Work out the finished part from the listing and answer in its coordinate system (mm). Face numbers are marked on the shaded views. A direction names the side the tool comes from. Round coordinates to 2 decimals unless told otherwise and drop trailing zeros. Order: outer loops, then holes, each group sorted by start corner. A loop starts at its lowest first (then second) coordinate and runs counter-clockwise, first axis right, second up. Notation, with made-up numbers: (27.25, 68.5) -> (38.25, 68.5) arc R20 cw to (38.25, 99.5) -> close; hole circle Ø6 at (-10.5, 87.25). An arc over 180 degrees is marked (long way). Use a Markdown table: item, result. Add a question column.
Item 1: Flat-ended cylindrical pins translate along their axes: P1, Ø6.5, axis at y = 44, z = 4, coming from the +X side; P2, Ø22.5, axis at x = 6.5, y = 19, coming from the -Z side; P3, Ø11, axis at y = 5.5, z = 5, coming from the +X side. Find the tip coordinate at first contact, or state that the pin passes through.
Item 2: A cutting plane is placed at C-C, the plane z = 2. Determine the outline of the cut face in (x, y), plus the area to 3 significant figures.
Item 3: For a pull along X with two mould halves and no side action, classify the marked faces 1, 2 and 3 as +X half, -X half, draft (parallel to the pull), parting line (faces both ways), or undercut.
Item 4: A tool of negligible diameter and unlimited length cuts with its end or side. For the marked faces 4, 5 and 6, from which of +Z, -Z, +X, -X, +Y, -Y can it reach the whole face along a straight path? Write none if from no direction.
Item 5: A cutting plane is placed at A-A, the plane y = 42. Give the number of separate pieces and of enclosed holes in the cut face, plus the area to 3 significant figures.
Item 6: A cutting plane is placed at B-B, the plane x = 65.75. Determine the outline of the cut face in (y, z).
Item 7: Find the intervals of material crossed by L1, parallel to Y at x = 65.75, z = -11; L2, parallel to Y at x = 10, z = -8.5; L3, parallel to X at y = 20, z = 7.25, in increasing order. Write a range as [from, to].
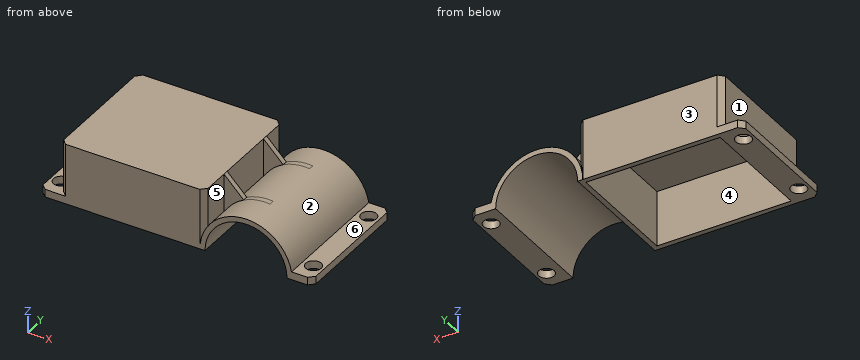
Autodesk Inventor part; units mm, degrees
ref_plane "YZ Plane" through (0, 0, 0) normal (1, 0, 0) x (0, 1, 0)
ref_plane "XZ Plane" through (0, 0, 0) normal (0, 1, 0) x (-1, 0, 0)
ref_plane "XY Plane" through (0, 0, 0) normal (0, 0, 1) x (1, 0, 0)
sketch "Esboço1" plane through (0, 0, 0) normal (0, 1, 0) x (-1, 0, 0)
  line L0 (-28, -11.75) -> (28, -11.75)
  line L1 (28, -11.75) -> (28, 11.75)
  line L2 (28, 11.75) -> (-28, 11.75)
  line L3 (-28, 11.75) -> (-28, -11.75)
  line L4 (-28, -11.75) -> (28, 11.75) construction
  line L5 (28, -11.75) -> (-28, 11.75) construction
  point P0 (0, 0)
  dimension "d0" = 56
  dimension "d1" = 23.5
extrude "Extrusão1" add sketch "Esboço1" along normal blind 49
sketch "Esboço2" plane through (28, 0, -11.75) normal (0, 0, -1) x (-1, 0, 0)
  line L0 (0, 49) -> (56, 49)
  line L1 (0, 49) -> (-33.75, 49)
  line L2 (-33.75, 49) -> (-33.75, 0)
  line L3 (0, 0) -> (56, 0)
  line L4 (-33.75, 0) -> (0, 0)
  line L5 (0, 0) -> (0, 49)
  point P0 (28, 0)
  dimension "d4" = 33.75
extrude "Extrusão2" add sketch "Esboço2" against normal blind 17.875
sketch "Esboço3" plane through (0, 49, 0) normal (0, 1, 0) x (1, 0, 0)
  line L0 (-28, 11.75) -> (61.75, 11.75)
  line L1 (61.75, 11.75) -> (59.75, 11.75)
  line L2 (59.75, 11.75) -> (43.875, 11.75)
  circle A0 centre (43.875, 11.75) radius 15.875
  point P0 (0, 0)
  dimension "d7" = 2
  dimension "d8" = 15.875
extrude "Extrusão3" cut sketch "Esboço3" against normal blind 49
sketch "Esboço4" plane through (61.75, 0, -11.75) normal (0, 0, -1) x (-1, 0, 0)
  line L0 (0, 49) -> (33.75, 49)
  line L1 (33.75, 0) -> (0, 0)
  line L2 (0, 49) -> (0, 0)
  line L3 (0, 0) -> (-8, 0)
  line L4 (-8, 0) -> (-8, 49)
  line L5 (-8, 49) -> (0, 49)
  line L6 (-4, 0) -> (-4, 7)
  line L7 (-4, 49) -> (-4, 42)
  circle A0 centre (-4, 42) radius 3
  circle A1 centre (-4, 7) radius 3
  point P0 (61.75, 0)
  dimension "d11" = 8
  dimension "d12" = 7
  dimension "d13" = 7
  dimension "d14" = 6
  dimension "d15" = 6
extrude "Extrusão4" add sketch "Esboço4" against normal blind 3
sketch "Esboço5" plane through (0, 49, 0) normal (0, 1, 0) x (1, 0, 0)
  arc A0 (28, 11.75) -> (59.75, 11.75) centre (43.875, 11.75) ccw
  circle A1 centre (43.875, 11.75) radius 17.875
  line L0 (61.75, -6.125) -> (28, -6.125)
  line L1 (69.75, 8.75) -> (61.75, 8.75)
  line L2 (61.75, 8.75) -> (61.4965, 8.75)
  line L3 (61.75, 8.75) -> (61.75, -6.125)
  line L4 (43.875, -6.125) -> (61.75, -6.125)
  line L5 (28, -11.75) -> (28, -6.125)
  line L6 (43.875, -6.125) -> (28, -6.125)
  line L7 (28, -6.125) -> (28, 3.5342)
  point P0 (0, 0)
extrude "Extrusão5" cut sketch "Esboço5" against normal blind 49 contours A1 L0 L7 | L2 L3 L0 A1
sketch "Esboço6" plane through (-28, 0, -11.75) normal (0, 0, -1) x (-1, 0, 0)
  line L0 (0, 0) -> (0, 49)
  line L1 (0, 49) -> (0, 0)
  line L2 (0, 0) -> (8, 0)
  line L3 (8, 0) -> (8, 49)
  line L4 (8, 49) -> (0, 49)
  line L5 (4, 49) -> (4, 42)
  line L6 (4, 0) -> (4, 7)
  circle A0 centre (4, 7) radius 3
  circle A1 centre (4, 42) radius 3
  point P0 (-28, 0)
  dimension "d20" = 8
  dimension "d21" = 7
  dimension "d22" = 7
  dimension "d23" = 6
  dimension "d24" = 6
extrude "Extrusão6" add sketch "Esboço6" against normal blind 3
sketch "Esboço8" plane through (28, 0, -11.75) normal (0, 0, -1) x (-1, 0, 0)
  line L0 (0, 49) -> (0, 0)
  line L1 (0, 49) -> (0, 47)
  line L2 (0, 47) -> (2, 47)
  line L3 (2, 47) -> (2, 2)
  line L4 (2, 47) -> (47, 47) construction
  line L5 (2, 2) -> (54, 2)
  line L6 (2, 2) -> (54, 2) construction
  line L7 (54, 2) -> (54, 47)
  line L8 (54, 47) -> (2, 47)
  point P0 (28, 0)
  dimension "d27" = 2
  dimension "d28" = 2
  dimension "d29" = 45
  dimension "d30" = 90
  dimension "d31" = 52
  dimension "d32" = 0
extrude "Extrusão7" cut sketch "Esboço8" against normal blind 21.5
sketch "Esboço10" plane through (28, 0, 11.75) normal (1, 0, 0) x (0, 0, -1)
  line L0 (0, 0) -> (0, 49)
  line L1 (0, 49) -> (0, 37)
  line L2 (0, 0) -> (0, 12)
  line L3 (0, 12) -> (16, 12)
  line L4 (16, 12) -> (16, 14)
  line L5 (16, 14) -> (0, 14)
  line L6 (0, 12) -> (0, 14)
  line L7 (0, 37) -> (16, 37)
  line L8 (16, 37) -> (16, 39)
  line L9 (16, 39) -> (0, 39)
  point P0 (11.75, 0)
  dimension "d38" = 12
  dimension "d41" = 12
  dimension "d42" = 16
  dimension "d43" = 2
  dimension "d44" = 16
  dimension "d45" = 2
extrude "Extrusão9" add sketch "Esboço10" along normal blind 17.875
sketch "Esboço11" plane through (28, 39, 11.75) normal (0, 1, 0) x (1, 0, 0)
  arc A0 (0, 15.2842) -> (33.4965, 20.5) centre (15.875, 23.5) ccw
  arc A1 (0, 23.5) -> (31.75, 23.5) centre (15.875, 23.5) ccw
  line L0 (17.875, 0) -> (17.875, 5.7372)
  line L1 (17.875, 5.7372) -> (17.875, 0)
  line L2 (0, 0) -> (17.875, 0)
  line L3 (17.875, 0) -> (0, 0)
  line L4 (0, 0) -> (7.6367, 7.6367)
  arc A2 (0, 15.2842) -> (17.875, 5.7372) centre (15.875, 23.5) ccw
  arc A3 (7.6367, 7.6367) -> (17.875, 5.7372) centre (15.875, 23.5) ccw
  line L5 (1.8834, 16) -> (17.875, 16)
  line L6 (1.8834, 16) -> (17.875, 16)
  line L7 (17.875, 16) -> (17.875, 7.7515)
  line L8 (17.875, 16) -> (17.875, 7.7515)
  arc A4 (1.8834, 16) -> (17.875, 7.7515) centre (15.875, 23.5) ccw
  point P0 (-28, 11.75)
  dimension "d48" = 45
extrude "Extrusão10" cut sketch "Esboço11" against normal blind 27.875
chamfer "Chanfro1" distance 2 angle 45 8 edges at (28, 49, 4.1079) (28, 0, 4.1079) (-28, 0, 1.5) (-28, 49, 1.5) (69.75, 49, -10.25) (69.75, 0, -10.25) (-36, 49, -10.25) (-36, 0, -10.25)
properties part number "KS  Dianteiro Front"
Reported:
| question | item | result |
|---|---|---|
| 1 | P1 | x = 56.65 |
| 1 | P2 | z = 9.75 |
| 1 | P3 | x = 57.77 |
| 2 | outline | (-28, 2) -> (-26, 0) -> (26, 0) -> (28, 2) -> (28, 12) -> (32.45, 12) -> (32.45, 0) -> (35.94, 0) -> (35.94, 49) -> (32.45, 49) -> (32.45, 39) -> (28, 39) -> (28, 47) -> (26, 49) -> (-26, 49) -> (-28, 47) -> close; (51.81, 0) -> (55.3, 0) -> (55.3, 49) -> (51.81, 49) -> close; hole (-26, 2) -> (26, 2) -> (26, 47) -> (-26, 47) -> close; hole (28, 14) -> (32.45, 14) -> (32.45, 37) -> (28, 37) -> close |
| 2 | area | 756 mm² |
| 3 | face 1 | -X half |
| 3 | face 2 | undercut |
| 3 | face 3 | draft |
| 4 | face 4 | -Z |
| 4 | face 5 | +Z, -Y |
| 4 | face 6 | +Z, +X, +Y, -Y |
| 5 | separate pieces | 3 |
| 5 | enclosed holes | 0 |
| 5 | area | 305 mm² |
| 6 | outline | (0, -11.75) -> (4, -11.75) -> (4, -8.75) -> (0, -8.75) -> close; (10, -11.75) -> (39, -11.75) -> (39, -8.75) -> (10, -8.75) -> close; (45, -11.75) -> (49, -11.75) -> (49, -8.75) -> (45, -8.75) -> close |
| 7 | L1 | [0, 4], [10, 39], [45, 49] |
| 7 | L2 | [0, 2], [47, 49] |
| 7 | L3 | [-28, -26], [26, 28] |
